Could you check a few things on this model? Use its own coordinates, in mm. Face numbers are marked on the shaded views. A direction names the side the tool comes from. Coordinates: 2 decimals unless noted, no trailing zeros. Loops run counter-clockwise (first coordinate to the right, second up) from the corner with the lowest first, then second, coordinate; pieces in that order, holes last.
1) Will these pins go through, and if not, where does the flat tip stop? P1, Ø7, axis at x = 3, y = 10, coming from the +Z side; P2, Ø1.5, axis at x = -3.5, z = 9, coming from the -Y side; P3, Ø1, axis at x = -6, z = 2, coming from the +Y side.
2) If I drill on line 1 along Y through (x, z) = (-2, 3); line 2 along Y through (x, z) = (-1.5, 3); line 3 along Z through (x, y) = (1.25, 8), over which ranges is the centre line in solid material (lowest first)?
3) Imagine slicing it at B-B on y = 12. Please give me the cut outline in (x, z).
4) Thinking about a two-plate mould opening in X: for the marked faces 4, 5 and 6, which applies, released by +X, released by -X, zero draft, split by the parting line, or undercut?
5) Imagine slicing it at A-A on z = 3. Please give me the cut outline in (x, y), plus the area to 3 significant figures.
6) Imagine slicing it at C-C on z = 9. Please give me the cut outline in (x, y).
7) For the marked faces 1, 2 and 3, which set-ups out of +Z, -Z, +X, -X, +Y, -Y let a thin tool reach every point of the face, with its end or its side?
8) Imagine slicing it at D-D on x = -4.25. Please give me the cut outline in (y, z), plus the area to 3 significant figures.
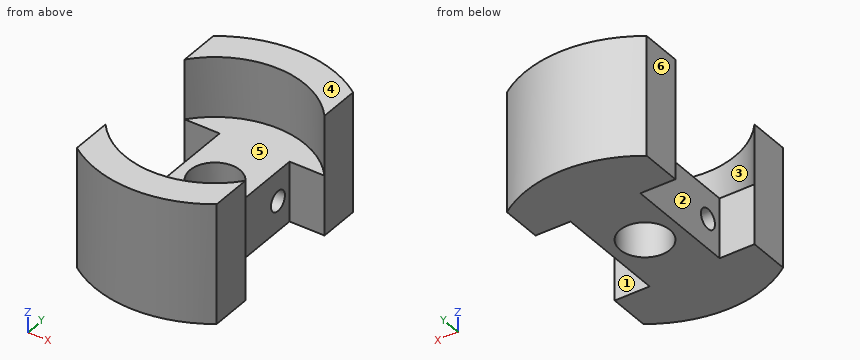
Autodesk Inventor part; units mm, degrees
ref_plane "YZ Plane" through (0, 0, 0) normal (1, 0, 0) x (0, 1, 0)
ref_plane "XZ Plane" through (0, 0, 0) normal (0, 1, 0) x (-1, 0, 0)
ref_plane "XY Plane" through (0, 0, 0) normal (0, 0, 1) x (1, 0, 0)
sketch "Sketch1" plane through (0, 0, 0) normal (0, 0, 1) x (1, 0, 0)
  arc A0 (7, 17.6569) -> (-7, 17.6569) centre (0, 12) ccw
  arc A1 (7, 21.7468) -> (-7, 21.7468) centre (0, 12) ccw
  line L0 (-7, 17.6569) -> (-7, 21.7468)
  line L1 (7, 17.6569) -> (7, 21.7468)
  line L2 (-7, 17.6569) -> (-3.5, 17.6569)
  line L3 (-3.5, 17.6569) -> (-3.5, 6.3431)
  line L4 (-3.5, 6.3431) -> (-7, 6.3431)
  line L5 (-7, 6.3431) -> (-7, 2.2532)
  arc A2 (-7, 2.2532) -> (7, 2.2532) centre (0, 12) ccw
  arc A3 (-7, 6.3431) -> (7, 6.3431) centre (0, 12) ccw
  line L6 (7, 6.3431) -> (7, 2.2532)
  line L7 (7, 6.3431) -> (3.5, 6.3431)
  line L8 (3.5, 6.3431) -> (3.5, 17.6569)
  line L9 (3.5, 17.6569) -> (7, 17.6569)
  line L10 (0, 0) -> (0, 24) construction
  line L11 (-10.3169, 12) -> (3.5, 12) construction
  point P0 (0, 3)
  dimension "d4" = 24
  dimension "d5" = 12
  dimension "d6" = 14
  dimension "d7" = 9
  dimension "d8" = 3.5
  dimension "d9" = 12
  dimension "d10" = 7
  dimension "d11" = 3.5
  dimension "d12" = 9
  dimension "d13" = 12
extrude "Extrusion1" add sketch "Sketch1" along normal blind 6 contours L9 L8 L7 A3 L4 L3 L2 A0
extrude "Extrusion2" add sketch "Sketch1" along normal blind 12 contours A0 L0 A1 L1 | L6 A2 L5 A3
sketch "Sketch2" plane through (0, 0, 6) normal (0, 0, 1) x (1, 0, 0)
  circle A0 centre (0, 12) radius 2.5
  arc A1 (-7, 2.2532) -> (7, 2.2532) centre (0, 12) ccw
  point P0 (0, 0)
  point P1 (0, 0)
  point P2 (0, 0)
  dimension "d18" = 12
  dimension "d19" = 5
extrude "Extrusion3" cut sketch "Sketch2" against normal up to surface (6 mm away)
thread "Thread1"
sketch "Sketch3" plane through (3.5, 6.3431, 0) normal (1, 0, 0) x (0, 0, -1)
  line L0 (0, 0) -> (0, 11.3137)
  point P0 (0, -6.3431)
  point P1 (-3, 1.6569)
  point P2 (-3, 9.6569)
  point P3 (0, 5.6569)
  dimension "d24" = 3
  dimension "d25" = 8
  dimension "d26" = 4
hole "Hole1" at (3.5, 8, 3) at (3.5, 16, 3) direction (-1, 0, 0) diameter 2 depth 7
equation "\"d9\" = 0.5 * d4"
properties part number "42"
Filled in:
1. P1: stops at z = 6
1. P2: stops at y = 0.32
1. P3: stops at y = 22.67
2. line 1: y = 0.17 to 7, 9 to 10.5, 13.5 to 15, 17 to 23.83
2. line 2: y = 0.09 to 7, 9 to 10, 14 to 15, 17 to 23.91
2. line 3: z = 0 to 2, 4 to 6
3. outline: (-3.5, 0) - (-2.5, 0) - (-2.5, 6) - (-3.5, 6) - close; (2.5, 0) - (3.5, 0) - (3.5, 6) - (2.5, 6) - close
4. face 4: zero draft
4. face 5: undercut
4. face 6: released by -X
5. outline: (-7, 2.25) arc R12 ccw to (7, 2.25) - (7, 6.34) - (3.5, 6.34) - (3.5, 7) - (-3.5, 7) - (-3.5, 6.34) - (-7, 6.34) - close; (-7, 17.66) - (-3.5, 17.66) - (-3.5, 17) - (3.5, 17) - (3.5, 17.66) - (7, 17.66) - (7, 21.75) arc R12 ccw to (-7, 21.75) - close; (-3.5, 9) - (3.5, 9) - (3.5, 15) - (-3.5, 15) - close; hole circle Ø5 at (0, 12)
5. area: 189 mm2
6. outline: (-7, 2.25) arc R12 ccw to (7, 2.25) - (7, 6.34) arc R9 cw to (-7, 6.34) - close; (-7, 17.66) arc R9 cw to (7, 17.66) - (7, 21.75) arc R12 ccw to (-7, 21.75) - close
7. face 1: +Z, -Z, +X
7. face 2: +Z, -Z, -X
7. face 3: +Z
8. outline: (0.78, 0) - (6.34, 0) - (6.34, 6) - (4.07, 6) - (4.07, 12) - (0.78, 12) - close; (17.66, 0) - (23.22, 0) - (23.22, 12) - (19.93, 12) - (19.93, 6) - (17.66, 6) - close
8. area: 106 mm2
